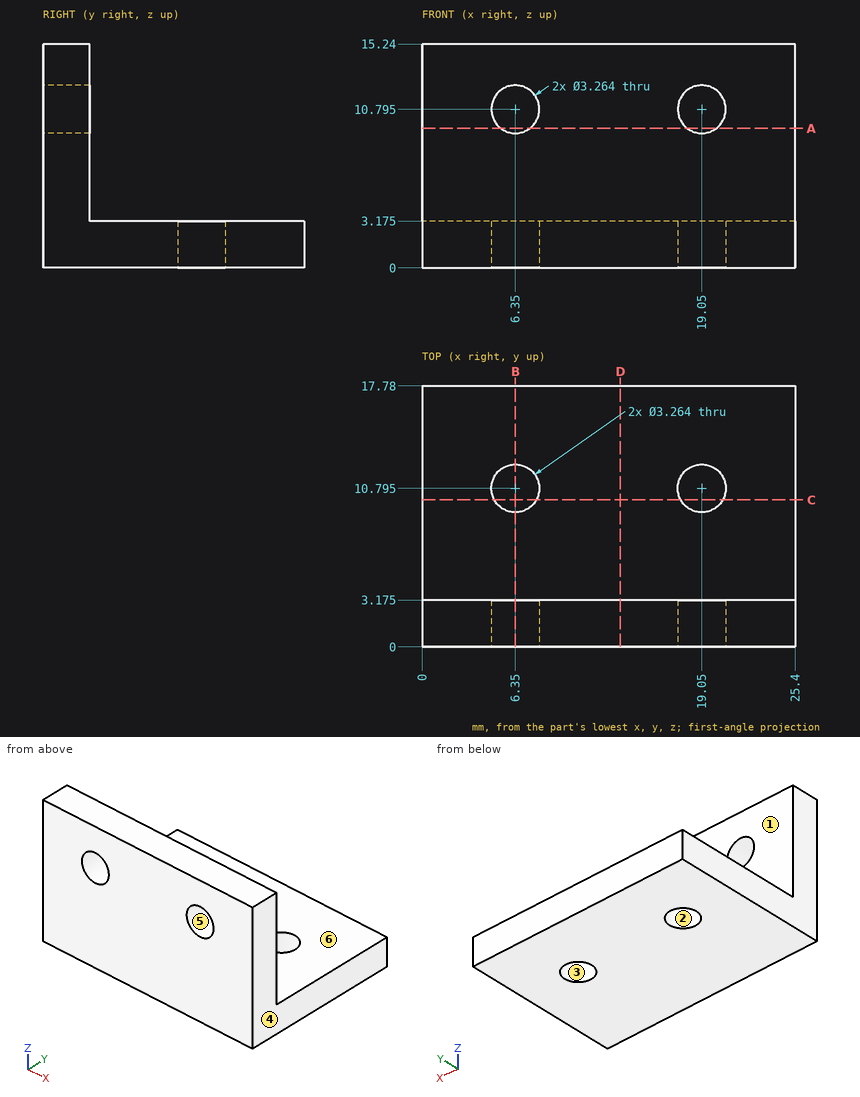
Could you check a few things on this drawing? It's one solid part, dimensions in mm from its lowest x, y, z. A direction names the side the tool comes from. Round coordinates to 2 decimals unless told otherwise and drop trailing zeros. Loops run counter-clockwise (first coordinate to the right, second up) from the corner with the lowest first, then second, coordinate; pieces in that order, holes last.
Q1. I want a section at D-D (x = 13.5). Write out the boundary of the cut face in (y, z) (3 decimals).
Q2. For P1, Ø2.5, axis at x = 6.35, z = 10.795, coming from the -Y side; P2, Ø6, axis at x = 17, z = 11.5, coming from the +Y side (3 decimals); P3, Ø5, axis at x = 6.35, y = 10.795, coming from the +Z side (3 decimals), each with a flat end and sliding along its axis, tell me the tip position at first contact or that it passes through.
Q3. Thinking about a two-plate mould opening in X: for the marked faces 1, 2, 3 and 4, which applies, pulls with the +X half, pulls with the -X half, needs draft (parallel to the pull), parting line crosses it, or undercut?
Q4. On a 3-axis mill with a long thin cutter (end or side, diameter ignored), from which of +Z, -Z, +X, -X, +Y, -Y can I reach the whole of each face in a straight line? I mean the marked faces 5 and 6. Say none if no direction works.
Q5. I want a section at B-B (x = 6.35). Write out the boundary of the cut face in (y, z) (3 decimals).
Q6. I want a section at A-A (z = 9.5). Write out the boundary of the cut face in (x, y) (3 decimals).
Q7. Please list where these lines run through material, in increasing order: L1, parallel to Z at x = 19.05, y = 1.85; L2, parallel to Y at x = 19.05, z = 2.4; L3, parallel to Z at x = 24, y = 3.25 (3 decimals).
Q8. I want a section at C-C (y = 10). Write out the boundary of the cut face in (x, z) (3 decimals).
Answer below:
1. outline: (0, 0) - (17.78, 0) - (17.78, 3.175) - (3.175, 3.175) - (3.175, 15.24) - (0, 15.24) - close
2. P1: passes through
2. P2: stops at y = 3.175
2. P3: stops at z = 3.175
3. face 1: needs draft
3. face 2: undercut
3. face 3: undercut
3. face 4: pulls with the +X half
4. face 5: +Y, -Y
4. face 6: +Z, +X, -X, +Y
5. outline: (0, 0) - (9.163, 0) - (9.163, 3.175) - (3.175, 3.175) - (3.175, 9.163) - (0, 9.163) - close; (0, 12.427) - (3.175, 12.427) - (3.175, 15.24) - (0, 15.24) - close; (12.427, 0) - (17.78, 0) - (17.78, 3.175) - (12.427, 3.175) - close
6. outline: (0, 0) - (5.357, 0) - (5.357, 3.175) - (0, 3.175) - close; (7.343, 0) - (18.057, 0) - (18.057, 3.175) - (7.343, 3.175) - close; (20.043, 0) - (25.4, 0) - (25.4, 3.175) - (20.043, 3.175) - close
7. L1: z = 0 to 9.16, 12.43 to 15.24
7. L2: y = 0 to 9.16, 12.43 to 17.78
7. L3: z = 0 to 3.175
8. outline: (0, 0) - (4.925, 0) - (4.925, 3.175) - (0, 3.175) - close; (7.775, 0) - (17.625, 0) - (17.625, 3.175) - (7.775, 3.175) - close; (20.475, 0) - (25.4, 0) - (25.4, 3.175) - (20.475, 3.175) - close
